Part print with two shaded views. Sizes in mm from the minimum x, y, z corner. A direction names the side the tool comes from. Round coordinates to 2 decimals unless told otherwise and drop trailing zeros. Write each loop counter-clockwise with the first axis right and the second up, starting at its lowest first coordinate (ties: lowest second). Pieces come first, ordered by that corner, then holes. Notation, with made-up numbers: (3.5, -11.75) -> (49.5, -11.75) arc R12 ccw to (49.5, 0.25) -> close; hole circle Ø4 at (-26.5, 15). An arc over 180 degrees is marked (long way). Put each result on its own line as item: value. Start each with the question number.
1. Saw through at A-A on x = 57.15. List the corners of the cut face in (y, z).
2. Saw through at B-B on y = 26. List the corners of the cut face in (x, z).
3. Saw through at C-C on z = 6.5. List the corners of the cut face in (x, y).
4. Saw through at D-D on x = 27. List the corners of the cut face in (y, z), and give its area (3 significant figures).
5. Pull direction X, two halves, no side cores. Call the marked faces 4, 5 and 6: pulls with the +X half, pulls with the -X half, needs draft (parallel to the pull), parting line crosses it, or undercut.
6. 3-axis set-ups, long thin cutter, end or side, ignore diameter. For the marked faces 1, 2 and 3: which of +Z, -Z, +X, -X, +Y, -Y reach the whole face in a straight line?
7. Flat gauge pins, fed straight in: P1, Ø21.5, axis at x = 84.5, y = 22.5, coming from the +Z side; P2, Ø16, axis at x = 59, z = 37.5, coming from the -Y side; P3, Ø2, axis at x = 26.5, z = 11.5, coming from the -Y side. Where does each tip first touch, or does it go through?
8. Drill centre lines: line 1 (Z direction, x = 41, y = 25); line 2 (Y direction, x = 71, z = 49); line 3 (Z direction, x = 13.5, y = 6.5). Where is each one in solid material? Low to high. Write a range as from..to.
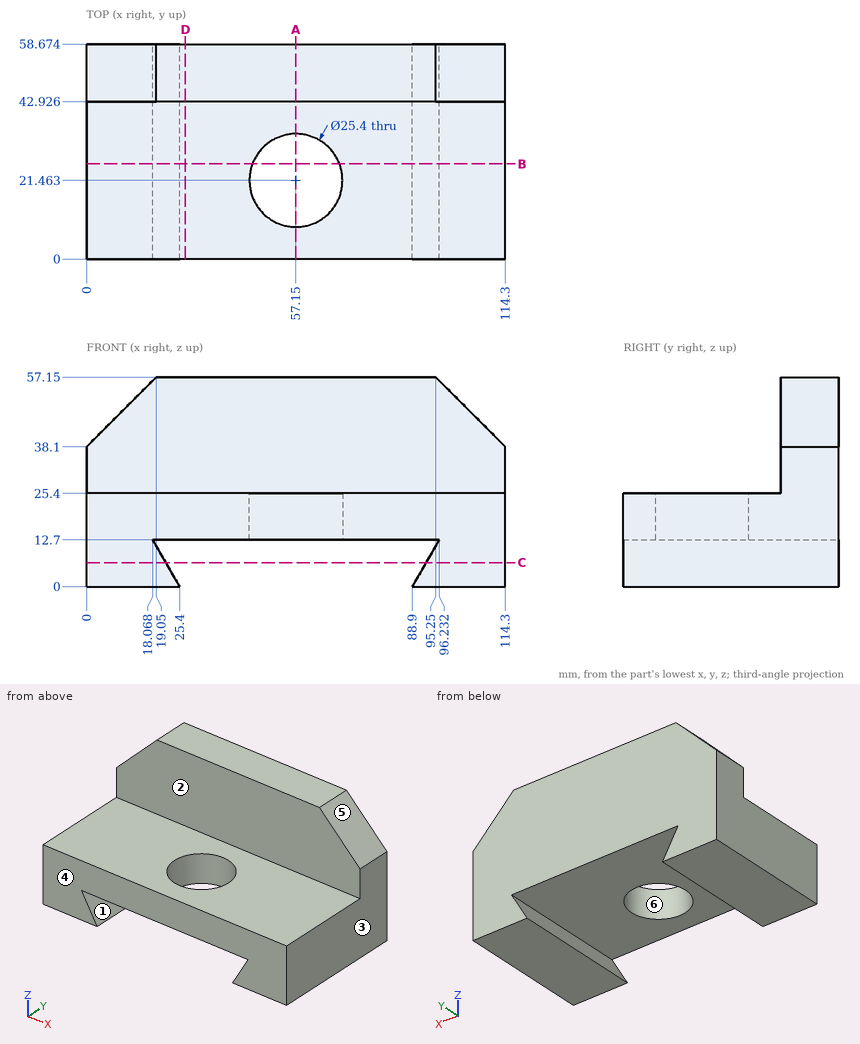
Return value:
1. outline: (0, 12.7) -> (8.76, 12.7) -> (8.76, 25.4) -> (0, 25.4) -> close; (34.16, 12.7) -> (58.67, 12.7) -> (58.67, 57.15) -> (42.93, 57.15) -> (42.93, 25.4) -> (34.16, 25.4) -> close
2. outline: (0, 0) -> (25.4, 0) -> (18.07, 12.7) -> (45.29, 12.7) -> (45.29, 25.4) -> (0, 25.4) -> close; (69.01, 12.7) -> (96.23, 12.7) -> (88.9, 0) -> (114.3, 0) -> (114.3, 25.4) -> (69.01, 25.4) -> close
3. outline: (0, 0) -> (21.65, 0) -> (21.65, 58.67) -> (0, 58.67) -> close; (92.65, 0) -> (114.3, 0) -> (114.3, 58.67) -> (92.65, 58.67) -> close
4. outline: (0, 12.7) -> (58.67, 12.7) -> (58.67, 57.15) -> (42.93, 57.15) -> (42.93, 25.4) -> (0, 25.4) -> close
4. area: 1,250 mm^2
5. face 4: needs draft
5. face 5: pulls with the +X half
5. face 6: undercut
6. face 1: +Y, -Y
6. face 2: +Z, +X, -X, -Y
6. face 3: +Z, -Z, +X, +Y, -Y
7. P1: stops at z = 25.4
7. P2: stops at y = 42.93
7. P3: passes through
8. line 1: z = 12.7..25.4
8. line 2: y = 42.93..58.67
8. line 3: z = 0..25.4
